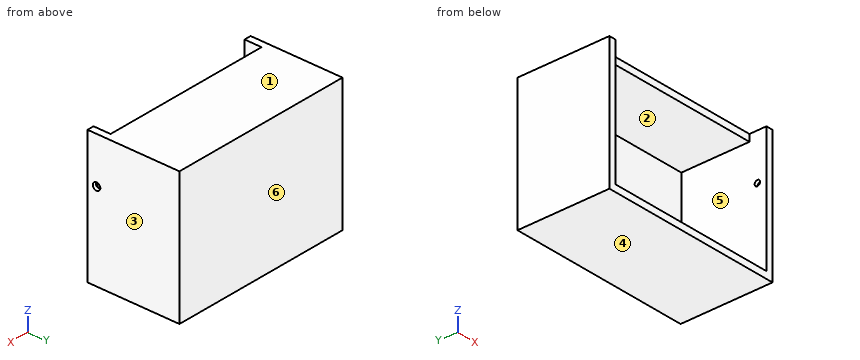
Autodesk Fusion 360 part; units mm, degrees
sketch "Sketch3" plane through (0, 106, 0) normal (0, 1, 0) x (-1, 0, 0)
  line L0 (0, -36) -> (0, 15)
  line L1 (0, 15) -> (-50, 15)
  line L2 (-50, 15) -> (-50, -36)
  line L3 (-50, -36) -> (0, -36)
  line L4 (0, -36) -> (-50, -36)
  line L5 (-50, -36) -> (-50, 0)
  line L6 (-50, 0) -> (0, 0)
  line L7 (0, 0) -> (0, -36)
  dimension "d1" = 36
sketch "Sketch1" plane through (0, 106, 0) normal (0, 1, 0) x (-1, 0, 0)
  line L0 (-50, 1) -> (0, 1)
  line L1 (0, 1) -> (0, -36)
  line L2 (0, -36) -> (-50, -36)
  line L3 (-50, -36) -> (-50, 1)
extrude "Extrude1" add sketch "Sketch1" along normal blind 22
extrude "Extrude2" add 1 faces at (50, 113.3333, -23.6667) along direction (1, 0, 0) blind 2
extrude "Extrude3" add 1 faces at (0, 113.3333, -11.3333) along direction (-1, 0, 0) blind 2
extrude "Extrude4" add 1 faces at (16, 113.3333, -36) along direction (0, 0, -1) blind 2
extrude "Extrude5" add 1 faces at (34, 106, -25) along direction (0, -1, 0) blind 5
shell "Shell1" thickness 2 removed faces 1 at (34, 101, -25)
sketch "Sketch2" plane through (0, 101, 0) normal (0, -1, 0) x (1, 0, 0)
  line L0 (50, -36) -> (0, -36)
  line L1 (0, -36) -> (0, -1)
  line L2 (0, -1) -> (50, -1)
  line L3 (50, -1) -> (50, -36)
  line L4 (52, -38) -> (52, 1)
  line L5 (52, 1) -> (-2, 1)
  line L6 (-2, 1) -> (-2, -38)
  line L7 (-2, -38) -> (52, -38)
  line L8 (0, 1) -> (50, 1)
  line L9 (50, 1) -> (50, -1)
  line L10 (50, -1) -> (0, -1)
  line L11 (0, -1) -> (0, 1)
extrude "Extrude6" cut sketch "Sketch2" against normal blind 5 contours L2 L5 L8 L9 L10 L11
hole "Hole1" at (52, 103.6557, -12.4599) direction (-1, 0, 0) diameter 1.623 depth 26 tip angle 118 counterbore diameter 2.2 counterbore depth 1
ref_plane "WorkPlane1" through (25, 114.5, -18.5) normal (1, 0, 0) x (0, 0, -1)
hole "Hole2" [suppressed]
hole "Hole3" [suppressed]
Can you work these out from the model? Positions are in its coordinate system, mm. Face numbers are marked on the shaded views. A direction names the side the tool comes from. Give positions to 0.01 mm unless a question says otherwise; leave off trailing zeros. Write each loop counter-clockwise with the first axis right and the second up, starting at its lowest first coordinate (ties: lowest second). Pieces come first, ordered by that corner, then holes. Notation, with made-up numbers: (38.5, 59.25) - (50.5, 59.25) arc R17 ccw to (50.5, 64.25) - close; hole circle Ø6 at (52, -37.75). An arc over 180 degrees is marked (long way). Write item = value, one per line. Start each with the question number.
1. For pin 1 (2.5 mm diameter, centred on y = 103.5, z = -12.5, fed in from +X); pin 2 (2 mm diameter, centred on x = 34, z = -0.5, fed in from -Y); pin 3 (1.9 mm diameter, centred on y = 103.66, z = -12.46, fed in from +X); pin 4 (4 mm diameter, centred on x = 22.5, z = -29, fed in from -Y), each with a flat end and sliding along its axis, tell me the tip position at first contact or that it passes through.
2. Thinking about a two-plate mould opening in Z: for the marked faces 1, 2, 3 and 4, which applies, released by +Z, released by -Z, zero draft, split by the parting line, or undercut?
3. Imagine slicing it at C-C (z = -29.5). Please give me the cut outline in (x, y).
4. On a 3-axis mill with a long thin cutter (end or side, diameter ignored), from which of +Z, -Z, +X, -X, +Y, -Y can I reach the whole of each face in a straight line? I mean the marked faces 5 and 6. Say none if no direction works.
5. Please list where these lines run through material, in increasing order: line 1 (X direction, y = 121.25, z = -17.5); line 2 (Z direction, x = 13.5, y = 106.75); line 3 (Y direction, x = 31.5, z = -24).
6. Imagine slicing it at A-A (y = 114.25). Please give me the cut outline in (x, z).
7. Imagine slicing it at D-D (x = 45.5). Please give me the cut outline in (y, z), and give its area (3 significant figures).
8. Imagine slicing it at B-B (z = -12.5). Please give me the cut outline in (x, y).
Worked answers:
q1.pin_1 = 52
q1.pin_2 = 106
q1.pin_3 = 51
q1.pin_4 = 126
q2.face_1 = released by +Z
q2.face_2 = undercut
q2.face_3 = zero draft
q2.face_4 = released by -Z
q3.outline = (-2, 101) - (0, 101) - (0, 126) - (50, 126) - (50, 101) - (52, 101) - (52, 128) - (-2, 128) - close
q4.face_5 = -Y
q4.face_6 = +Z, -Z, +X, -X, +Y
q5.line_1 = -2 to 0, 50 to 52
q5.line_2 = -38 to -36, -1 to 1
q5.line_3 = 126 to 128
q6.outline = (-2, -38) - (52, -38) - (52, 1) - (-2, 1) - close; hole (0, -36) - (50, -36) - (50, -1) - (0, -1) - close
q7.outline = (101, -38) - (128, -38) - (128, 1) - (106, 1) - (106, -1) - (126, -1) - (126, -36) - (101, -36) - close
q7.area = 168 mm2
q8.outline = (-2, 101) - (0, 101) - (0, 126) - (50, 126) - (50, 104.47) - (51, 104.47) - (51, 104.75) - (52, 104.75) - (52, 128) - (-2, 128) - close; (50, 101) - (52, 101) - (52, 102.56) - (51, 102.56) - (51, 102.85) - (50, 102.85) - close
